from build123d import *

# Parameters (mm, degrees)
SKETCH1_W                    = 49.765070753
SKETCH1_H                    = 64.93
BOSS_EXTRUDE1_DEPTH          = 2
BOSS_EXTRUDE1_TAPER          = 2
SKETCH3_R                    = 2
CUT_EXTRUDE2_DEPTH           = 2
CUT_EXTRUDE2_DRAFT           = -2
SKETCH4_W                    = 8
SKETCH4_H                    = 28.479841539
CUT_EXTRUDE3_DEPTH           = 2
CUT_EXTRUDE3_DRAFT           = -2
SKETCH4_H_2                  = 28.450158461
CUT_EXTRUDE3_PROFILE_2_DEPTH = 2
CUT_EXTRUDE3_PROFILE_2_DRAFT = -2


with BuildPart() as part:
    # Sketch1 → Boss-Extrude1 (new body)
    with BuildSketch(Plane.XY):
        with Locations((-98.472172046, 45.191977318)):
            Rectangle(SKETCH1_W, SKETCH1_H)
    extrude(amount=BOSS_EXTRUDE1_DEPTH, taper=BOSS_EXTRUDE1_TAPER)


with BuildPart() as cut_extrude2_tool:
    # Sketch3 → Cut-Extrude2 (with draft: the straight prism first)
    with BuildSketch(Plane.XY.offset(2)):
        with Locations((-119.284865883, 45.177135779)):
            Circle(SKETCH3_R)
    extrude(amount=-CUT_EXTRUDE2_DEPTH)
    # Cut-Extrude2: the draft: its side faces are tilted about the plane it starts from
    cut_extrude2_sides = [cut_extrude2_tool.faces().sort_by_distance(p)[0] for p in [
        (-121.284865883, 45.177135779, 1),
    ]]
    draft(cut_extrude2_sides, Plane.XY.offset(2), CUT_EXTRUDE2_DRAFT)


with BuildPart() as part_1:
    add(part.part)

    # Cut-Extrude2: cut by cut_extrude2_tool
    add(cut_extrude2_tool.part, mode=Mode.SUBTRACT)


with BuildPart() as cut_extrude3_tool:
    # Sketch4 → Cut-Extrude3 (with draft: the straight prism first)
    with BuildSketch(Plane(origin=(0, 0, 0), x_dir=(-1, 0, 0), z_dir=(0, 0, -1))):
        with Locations((119.354707422, 63.417056548)):
            Rectangle(SKETCH4_W, SKETCH4_H)
    extrude(amount=-CUT_EXTRUDE3_DEPTH)
    # Cut-Extrude3: the draft: its side faces are tilted about the plane it starts from
    cut_extrude3_sides = [cut_extrude3_tool.faces().sort_by_distance(p)[0] for p in [
        (-119.354707422, 77.656977318, 1),
        (-115.354707422, 63.417056548, 1),
        (-119.354707422, 49.177135779, 1),
        (-123.354707422, 63.417056548, 1),
    ]]
    draft(cut_extrude3_sides, Plane(origin=(0, 0, 0), x_dir=(-1, 0, 0), z_dir=(0, 0, -1)), CUT_EXTRUDE3_DRAFT)


with BuildPart() as part_2:
    add(part_1.part)

    # Cut-Extrude3: cut by cut_extrude3_tool
    add(cut_extrude3_tool.part, mode=Mode.SUBTRACT)


with BuildPart() as cut_extrude3_profile_2_tool:
    # Sketch4 → Cut-Extrude3 profile 2 (with draft: the straight prism first)
    with BuildSketch(Plane(origin=(0, 0, 0), x_dir=(-1, 0, 0), z_dir=(0, 0, -1))):
        with Locations((119.354707422, 26.952056549)):
            Rectangle(SKETCH4_W, SKETCH4_H_2)
    extrude(amount=-CUT_EXTRUDE3_PROFILE_2_DEPTH)
    # Cut-Extrude3 profile 2: the draft: its side faces are tilted about the plane it starts from
    cut_extrude3_profile_2_sides = [cut_extrude3_profile_2_tool.faces().sort_by_distance(p)[0] for p in [
        (-123.354707422, 26.952056548, 1),
        (-119.354707422, 41.177135779, 1),
        (-115.354707422, 26.952056548, 1),
        (-119.354707422, 12.726977318, 1),
    ]]
    draft(cut_extrude3_profile_2_sides, Plane(origin=(0, 0, 0), x_dir=(-1, 0, 0), z_dir=(0, 0, -1)), CUT_EXTRUDE3_PROFILE_2_DRAFT)


with BuildPart() as part_3:
    add(part_2.part)

    # Cut-Extrude3 profile 2: cut by cut_extrude3_profile_2_tool
    add(cut_extrude3_profile_2_tool.part, mode=Mode.SUBTRACT)


solid = part_3.part
Design review of the part built by this model. Coordinates are the model's own, in mm. Coordinates: 2 decimals unless noted, no trailing zeros. Loops run counter-clockwise (first coordinate to the right, second up) from the corner with the lowest first, then second, coordinate; pieces in that order, holes last. Notation, with made-up numbers: (-35.5, 18.25) -> (2.5, 18.25) arc R26 cw to (2.5, 41.25) -> close; hole circle Ø8 at (67, 31.5). An arc over 180 degrees is marked (long way). Use a Markdown table: item, result. Add a question column.
Item 1: We need section A-A, the plane z = 1.5. Write out the cut boundary in (x, y).
Item 2: Wall thickness on L1, parallel to Y at x = -87, z = 1.85; L2, parallel to X at y = 42.5, z = 1.55; L3, parallel to Y at x = -101.5, z = 0.45: over which ranges is each line inside the solid? List them lowest first. Write a range as from..to.
Item 3: We need section B-B, the plane y = 69.5. Write out the cut boundary in (x, z).
Item 4: The part is to be moulded in two halves that separate along X. For faces 1 (the flat face through (-93, 46, 2)), 2 (the conical face through (-121.25, 45.26, 1.01)), say which applies: +X half, -X half, draft (parallel to the pull), parting line (faces both ways), or undercut.
Numbers:
| question | item | result |
|---|---|---|
| 1 | outline | (-123.3, 41.12) -> (-115.41, 41.12) -> (-115.41, 12.78) -> (-73.64, 12.78) -> (-73.64, 77.6) -> (-115.41, 77.6) -> (-115.41, 49.23) -> (-123.3, 49.23) -> close; hole circle Ø3.97 at (-119.28, 45.18) |
| 2 | L1 | y = 12.79..77.59 |
| 2 | L2 | x = -123.3..-73.64 |
| 2 | L3 | y = 12.74..77.64 |
| 3 | outline | (-115.42, 2) -> (-115.35, 0) -> (-73.59, 0) -> (-73.66, 2) -> close |
| 4 | face 1 | draft |
| 4 | face 2 | undercut |
